Here's how the part is built. I have some questions about the finished solid (model axes, mm). Face numbers are marked on the shaded views. A direction names the side the tool comes from. Coordinates: 2 decimals unless noted, no trailing zeros. Write each loop counter-clockwise with the first axis right and the second up, starting at its lowest first coordinate (ties: lowest second). Pieces come first, ordered by that corner, then holes.
Item 1: For the marked faces 1, 2, 3, 4 and 5, which set-ups out of +Z, -Z, +X, -X, +Y, -Y let a thin tool reach every point of the face, with its end or its side?
Item 2: I want a section at C-C (x = -3). Please give me the cut outline in (y, z) (3 decimals), and give its area (3 significant figures).
Item 3: I want a section at D-D (x = 4.5). Please give me the cut outline in (y, z) (3 decimals), and give its area (3 significant figures).
Item 4: Please list where these lines run through material, in increasing order: line 1 (X direction, y = -3, z = 1.5); line 2 (Y direction, x = 5, z = 8.5) (3 decimals); line 3 (Z direction, x = -1, y = 4.25).
Item 5: I want a section at B-B (y = 3.25). Please give me the cut outline in (x, z), and give its area (3 significant figures).
Item 6: If we mould it in two halves opening along X, with no side actions, what happens to the marked faces 6, 7 and 8? For each: pulls with the +X half, pulls with the -X half, needs draft (parallel to the pull), parting line crosses it, or undercut.
Item 7: I'm going to push flat-ended pins straight in: P1, Ø1.1, axis at y = 0.5, z = 11, coming from the +X side; P2, Ø1, axis at x = 0, z = -6, coming from the -Y side; P3, Ø1.4, axis at x = -9, y = 0, coming from the -Z side. Where does each tip first touch, or does it pass through?
Item 8: I want a section at A-A (z = -9). Please give me the cut outline in (x, y), and give its area (3 significant figures).
from build123d import *

# Parameters (mm, degrees)
BOSS_EXTRUDE1_DEPTH      = 7.1
BOSS_EXTRUDE1_DEPTH_BACK = 7.1
FILLET1_R                = 3.5
BOSS_EXTRUDE2_DEPTH      = 1.25
BOSS_EXTRUDE2_DEPTH_BACK = 1.25


with BuildPart() as part:
    # Sketch1 → Boss-Extrude1 (new, two sides: drawn at the far end of the back side and taken through both)
    with BuildSketch(Plane(origin=(0, 0, 0), x_dir=(0, 0, -1), z_dir=(1, 0, 0)).offset(-BOSS_EXTRUDE1_DEPTH_BACK)):
        Polygon((11, -3.8), (11, 3.8), (0, 3.8), (0, 8), (-5, 8), (-5, 6.625), (-13.9, 6.625), (-16.9, 5.2), (-16.9, -5.2), (-13.9, -6.625), (-5, -6.625), (-5, -8), (0, -8), (0, -3.8), align=None)
    extrude(amount=BOSS_EXTRUDE1_DEPTH + BOSS_EXTRUDE1_DEPTH_BACK)

    # Fillet1
    fillet1_edges = [part.edges().sort_by_distance(p)[0] for p in [
        (0, -8, 0),
        (0, 8, 0),
        (7.1, 3.8, -5.5),
        (7.1, -3.8, -5.5),
        (-7.1, 3.8, -5.5),
        (-7.1, -3.8, -5.5),
    ]]
    fillet(fillet1_edges, radius=FILLET1_R)

    # Sketch2 → Boss-Extrude2 (add, two sides: drawn at the far end of the back side and taken through both)
    with BuildSketch(Plane(origin=(0, 0, 0), x_dir=(1, 0, 0), z_dir=(0, 1, 0)).offset(-BOSS_EXTRUDE2_DEPTH_BACK)):
        Polygon((-7.1, -16.9), (-9.7, -13.3), (-9.7, -11.9), (-8.4, -11.9), (-8.4, -10.5), (-7.1, -10.5), align=None)
        Polygon((7.1, -10.5), (7.1, -16.9), (9.7, -13.3), (9.7, -11.9), (8.4, -11.9), (8.4, -10.5), align=None)
    extrude(amount=BOSS_EXTRUDE2_DEPTH + BOSS_EXTRUDE2_DEPTH_BACK)


solid = part.part
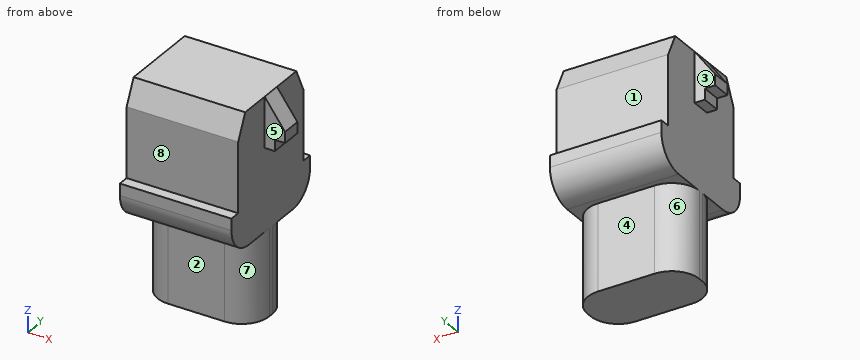
Answer:
1. face 1: +Z, +X, -X, +Y
1. face 2: -Z, +X, -X, -Y
1. face 3: +Z, -Z, -X, +Y
1. face 4: -Z, +X, -X, +Y
1. face 5: +Z, -Z, +X, -Y
2. outline: (-8, 3.5) arc R3.5 ccw to (-4.5, 0) - (-3.8, 0) - (-3.8, -11) - (3.8, -11) - (3.8, 0) - (4.5, 0) arc R3.5 ccw to (8, 3.5) - (8, 5) - (6.625, 5) - (6.625, 13.9) - (5.2, 16.9) - (-5.2, 16.9) - (-6.625, 13.9) - (-6.625, 5) - (-8, 5) - close
2. area: 312 mm2
3. outline: (-8, 3.5) arc R3.5 ccw to (-4.5, 0) - (-3.682, 0) - (-3.682, -11) - (3.682, -11) - (3.682, 0) - (4.5, 0) arc R3.5 ccw to (8, 3.5) - (8, 5) - (6.625, 5) - (6.625, 13.9) - (5.2, 16.9) - (-5.2, 16.9) - (-6.625, 13.9) - (-6.625, 5) - (-8, 5) - close
3. area: 309 mm2
4. line 1: x = -7.1 to 7.1
4. line 2: y = -6.625 to 6.625
4. line 3: z = 0 to 16.9
5. outline: (-7.1, 0) - (-5.48, 0) - (-5.48, -11) - (5.48, -11) - (5.48, 0) - (7.1, 0) - (7.1, 16.9) - (-7.1, 16.9) - close
5. area: 361 mm2
6. face 6: pulls with the -X half
6. face 7: pulls with the +X half
6. face 8: needs draft
7. P1: stops at x = 8.4
7. P2: stops at y = -3.8
7. P3: stops at z = 10.5
8. outline: (-7.1, -0.3) arc R3.5 ccw to (-3.6, -3.8) - (3.6, -3.8) arc R3.5 ccw to (7.1, -0.3) - (7.1, 0.3) arc R3.5 ccw to (3.6, 3.8) - (-3.6, 3.8) arc R3.5 ccw to (-7.1, 0.3) - close
8. area: 97.4 mm2
